```python
from build123d import *

# Parameters (mm, degrees)
F0_R     = 11.5
F1_DEPTH = 14
F2_R     = 9.5
F3_DEPTH = 5
F5_DEPTH = 8
F6_R     = 1
F7_DEPTH = 14.001
F9_DEPTH = 4


with BuildPart() as f1:
    # F0 (on Front) → F1 (new body)
    with BuildSketch(Plane.XZ):
        Circle(F0_R)
    extrude(amount=-F1_DEPTH)

    # F2 (on face) → F3 (cut)
    with BuildSketch(Plane.XZ):
        Circle(F2_R)
    extrude(amount=-F3_DEPTH, mode=Mode.SUBTRACT)

    # F4 (on face) → F5 (cut)
    with BuildSketch(Plane.XZ.offset(-5)):
        with BuildLine():
            Line((-2.481935, 0.3), (2.481935, 0.3))
            ThreePointArc((2.481935, 0.3), (0, 2.5), (-2.481935, 0.3))
        make_face()
        with BuildLine():
            Line((2.481935, -0.3), (-2.481935, -0.3))
            ThreePointArc((-2.481935, -0.3), (0, -2.5), (2.481935, -0.3))
        make_face()
    extrude(amount=-F5_DEPTH, mode=Mode.SUBTRACT)

    # F6 (on face) → F7 (cut, through all)
    with BuildSketch(Plane(origin=(0, 14, 0), x_dir=(-1, 0, 0), z_dir=(0, 1, 0))):
        with Locations((0, 12)):
            Circle(F6_R)
        with Locations((-2.984279, 11.622998)):
            Circle(F6_R)
        with Locations((-5.781044, 10.51568)):
            Circle(F6_R)
        with Locations((-8.214565, 8.747624)):
            Circle(F6_R)
        with Locations((-10.131935, 6.429922)):
            Circle(F6_R)
        with Locations((-11.412678, 3.708204)):
            Circle(F6_R)
        with Locations((-11.976321, 0.753486)):
            Circle(F6_R)
        with Locations((-11.787447, -2.248576)):
            Circle(F6_R)
        with Locations((-10.857925, -5.109351)):
            Circle(F6_R)
        with Locations((-9.246159, -7.649088)):
            Circle(F6_R)
        with Locations((-7.053423, -9.708204)):
            Circle(F6_R)
        with Locations((-4.417495, -11.157318)):
            Circle(F6_R)
        with Locations((-1.503999, -11.905376)):
            Circle(F6_R)
        with Locations((1.503999, -11.905376)):
            Circle(F6_R)
        with Locations((4.417495, -11.157318)):
            Circle(F6_R)
        with Locations((7.053423, -9.708204)):
            Circle(F6_R)
        with Locations((9.246159, -7.649088)):
            Circle(F6_R)
        with Locations((10.857925, -5.109351)):
            Circle(F6_R)
        with Locations((11.787447, -2.248576)):
            Circle(F6_R)
        with Locations((11.976321, 0.753486)):
            Circle(F6_R)
        with Locations((11.412678, 3.708204)):
            Circle(F6_R)
        with Locations((10.131935, 6.429922)):
            Circle(F6_R)
        with Locations((8.214565, 8.747624)):
            Circle(F6_R)
        with Locations((5.781044, 10.51568)):
            Circle(F6_R)
        with Locations((2.984279, 11.622998)):
            Circle(F6_R)
    extrude(amount=-F7_DEPTH, mode=Mode.SUBTRACT)

    # F8 (on face) → F9 (join)
    with BuildSketch(Plane.XZ):
        Polygon((8.67528, -9.12357), (10.587552, -6.81203), (8.661268, -5.21847), (6.748996, -7.53001), align=None)
    extrude(amount=-F9_DEPTH)


solid = f1.part
```
Input: part model. Units: mm. Frame: model coordinates. Coordinates: 2 decimals unless noted, no trailing zeros. Loops run counter-clockwise (first coordinate to the right, second up) from the corner with the lowest first, then second, coordinate; pieces in that order, holes last. Notation, with made-up numbers: M -15.5,85.5 L 37.5,85.5 A13 cw 37.5,109.5 Z; hole C 44.25,-8.5 d10. An arc over 180 degrees is marked long. Answer in a Markdown table with one row per item.
1. Section B-B, the plane y = 7.75. Count the separate pieces of the cut face and the enclosed holes in it, then the cut area to 3 significant figures.
Response:
| item | result |
|---|---|
| separate pieces | 1 |
| enclosed holes | 2 |
| area | 384 mm2 |
2. Draft query along X for faces 1 (the cylindrical face through (-7.878, 6.902, -8.377)), 2 (the cylindrical face through (8.87, 6.9, 7.32)), 3 (the cylindrical face through (-1.39, 7.1, -10.91)), 4 (the cylindrical face through (-0.1, 8.9, -2.5)). Return one class per face: pulls with the +X half, pulls with the -X half, needs draft (parallel to the pull), parting line crosses it, or undercut.
Response:
| item | result |
|---|---|
| face 1 | pulls with the -X half |
| face 2 | pulls with the +X half |
| face 3 | undercut |
| face 4 | undercut |
3. Section C-C, the plane x = 3. Output: boundary loops of the cut face in (y, z), then the cut area to 3 significant figures.
Response:
| item | result |
|---|---|
| outline | M 0,-11.1 L 14,-11.1 L 14,10.62 L 0,10.62 L 0,9.01 L 5,9.01 L 5,-9.01 L 0,-9.01 Z |
| area | 214 mm2 |
4. Section A-A, the plane x = 0. Output: boundary loops of the cut face in (y, z), then the cut area to 3 significant figures.
Response:
| item | result |
|---|---|
| outline | M 0,-11.5 L 14,-11.5 L 14,11 L 0,11 L 0,9.5 L 5,9.5 L 5,2.5 L 13,2.5 L 13,0.3 L 5,0.3 L 5,-0.3 L 13,-0.3 L 13,-2.5 L 5,-2.5 L 5,-9.5 L 0,-9.5 Z |
| area | 185 mm2 |
5. First-contact query: pin 1 (5 mm diameter, centred on x = -0.5, z = -6.5, fed in from -Y); pin 2 (5 mm diameter, centred on y = 7.5, z = -3, fed in from +X); pin 3 (1.5 mm diameter, centred on y = 9.5, z = -4.5, fed in from +X). Flat tips, straight axial feed; report the tip coordinate or a pass-through.
Response:
| item | result |
|---|---|
| pin 1 | stops at y = 5 |
| pin 2 | stops at x = 11.49 |
| pin 3 | stops at x = 10.87 |
6. Material intervals for line 1 (Z direction, x = 0, y = 2.6); line 2 (Y direction, x = -4.5, z = -7.5); line 3 (X direction, y = 11, z = 8.75), sorted ascending.
Response:
| item | result |
|---|---|
| line 1 | z = -11.5 to -9.5, 9.5 to 11 |
| line 2 | y = 5 to 14 |
| line 3 | x = -7.21 to 7.21 |
